Verification items for the finished model (mm, model axes). A direction names the side the tool comes from. Give positions to 0.01 mm unless a question says otherwise; leave off trailing zeros. Loops run counter-clockwise (first coordinate to the right, second up) from the corner with the lowest first, then second, coordinate; pieces in that order, holes last. Notation, with made-up numbers: M -20,-21.75 L 37,-21.75 A26 ccw 37,3.25 Z; hole C 62,-35.75 d3. An arc over 180 degrees is marked long. Put each result on its own line as item: value. Start each with the question number.
from build123d import *

# Parameters (mm, degrees)
F0_R     = 6.35
F0_W     = 25.4
F0_H     = 117.7036
F0_R_2   = 3.175
F1_DEPTH = 12.7


with BuildPart() as f1:
    # F0 (on Top) → F1 (new body)
    with BuildSketch(Plane.XY):
        Polygon((38.1, -12.7), (38.1, 12.7), (12.7, 12.7), (-12.7, 12.7), (-38.1, 12.7), (-38.1, -12.7), align=None)
        with Locations((-10.4775, 0)):
            Circle(F0_R, mode=Mode.SUBTRACT)
        with Locations((10.4775, 0)):
            Circle(F0_R, mode=Mode.SUBTRACT)
        with Locations((0, 71.5518)):
            Rectangle(F0_W, F0_H)
        with Locations((-6.35, 124.0536)):
            Circle(F0_R_2, mode=Mode.SUBTRACT)
        with Locations((6.35, 124.0536)):
            Circle(F0_R_2, mode=Mode.SUBTRACT)
    extrude(amount=F1_DEPTH)


solid = f1.part
Q1. Scan lines: L1, parallel to Y at x = 10, z = 8.75; L2, parallel to X at y = 122.5, z = 12.25; L3, parallel to Y at x = -7, z = 8.75. Record each from-to range of solid material in increasing order.
Q2. Cross-section at B-B, the plane z = 5. State how many separate pieces and enclosed holes the cut face has, then the cut area to 3 significant figures.
Q3. Set-up check for faces 1 (the face through (38.1, 0, 6)), 2 (the face through (26, 12.7, 6)), 3 (the face through (-12.7, 71, 6)): record each of +Z, -Z, +X, -X, +Y, -Y from which the full face is reachable in a straight line by a thin tool's end or side.
Q4. Cross-section at C-C, the plane x = -6.35. Record the boundary of the cut face in (y, z).
Q5. Cross-section at A-A, the plane y = 0. Record the boundary of the cut face in (x, z).
Q6. Go/stop test with flat-tipped pins: pin 1 (4 mm diameter, centred on x = 18, z = 2.5, fed in from +Y); pin 2 (4 mm diameter, centred on y = 57, z = 7.5, fed in from +X). Record where each tip stops, or that it passes through.
Q7. Cross-section at D-D, the plane x = -24. Record the boundary of the cut face in (y, z).
Q8. Release check for a two-part mould opening along X. For faces 4 (the face through (-1, 44, 12.7)), 5 (the face through (12.7, 71, 6)), 6 (the face through (4.134, 0.279, 6.261)), 7 (the face through (-38.1, 0, 6)) record: pulls with the +X half, pulls with the -X half, needs draft (parallel to the pull), parting line crosses it, or undercut.
Ans:
1. L1: y = -12.7 to -6.33, 6.33 to 130.4
1. L2: x = -12.7 to -9.12, -3.58 to 3.58, 9.12 to 12.7
1. L3: y = -12.7 to -5.31, 5.31 to 120.95, 127.16 to 130.4
2. separate pieces: 1
2. enclosed holes: 4
2. area: 4,610 mm^2
3. face 1: +Z, -Z, +X, +Y, -Y
3. face 2: +Z, -Z, +X, +Y
3. face 3: +Z, -Z, -X, +Y
4. outline: M -12.7,0 L -4.83,0 L -4.83,12.7 L -12.7,12.7 Z; M 4.83,0 L 120.88,0 L 120.88,12.7 L 4.83,12.7 Z; M 127.23,0 L 130.4,0 L 130.4,12.7 L 127.23,12.7 Z
5. outline: M -38.1,0 L -16.83,0 L -16.83,12.7 L -38.1,12.7 Z; M -4.13,0 L 4.13,0 L 4.13,12.7 L -4.13,12.7 Z; M 16.83,0 L 38.1,0 L 38.1,12.7 L 16.83,12.7 Z
6. pin 1: stops at y = 12.7
6. pin 2: stops at x = 12.7
7. outline: M -12.7,0 L 12.7,0 L 12.7,12.7 L -12.7,12.7 Z
8. face 4: needs draft
8. face 5: pulls with the +X half
8. face 6: undercut
8. face 7: pulls with the -X half
